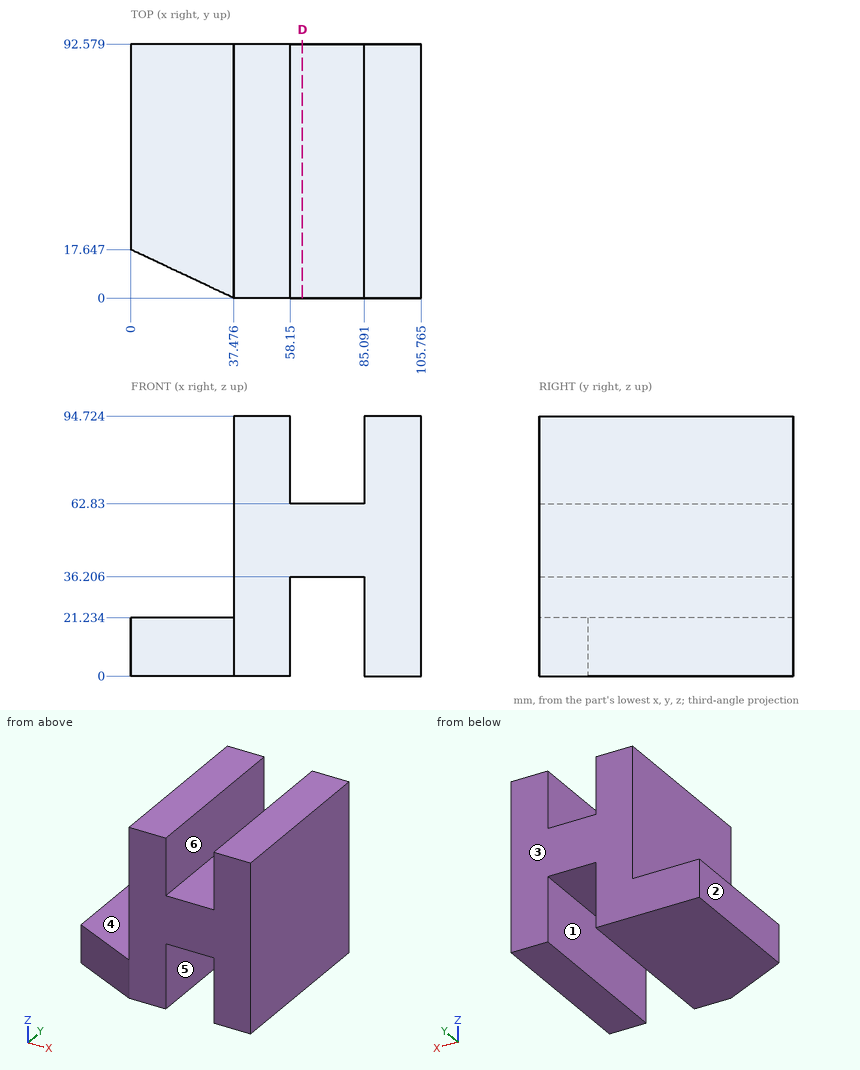
Print and shaded views of the part. All mm, measured from the part's lowest x, y and z. A direction names the side the tool comes from. Coordinates: 2 decimals unless noted, no trailing zeros. Order: outer loops, then holes, each group sorted by start corner. A loop starts at its lowest first (then second) coordinate and runs counter-clockwise, first axis right, second up. Notation, with made-up numbers: (28, -1) - (63, -1) arc R26 ccw to (63, 29) - close; hole circle Ø11 at (56.25, 43). An arc over 180 degrees is marked (long way). Return JSON: item names as keys, results as strings. Group by question number.
Item 1: Drill centre lines: probe 1 along Z at (x, y) = (58.5, 65) (1 decimal); probe 2 along X at (y, z) = (49, 55.5) (1 decimal); probe 3 along Z at (x, y) = (7.5, 83). Where is each one in solid material? Low to high. Write a range as from..to.
Item 2: Pin check, flat tips, straight feed: pin 1 (5 mm diameter, centred on y = 18.5, z = 41, fed in from -X); pin 2 (10 mm diameter, centred on x = 68.5, y = 23.5, fed in from -Z); pin 3 (13.5 mm diameter, centred on x = 66, y = 48.5, fed in from +Z). Stop position of each tip, or through.
Item 3: Which spindle directions (+Z, -Z, +X, -X, +Y, -Y) get a long thin tool onto all of the face, cutting with end or side? Do the marked faces 4, 5 and 6. Say none if no direction does.
Item 4: Pull direction X, two halves, no side cores. Call the marked faces 1, 2 and 3: pulls with the +X half, pulls with the -X half, needs draft (parallel to the pull), parting line crosses it, or undercut.
Item 5: Cut at D-D (x = 62.5). List the corners of the cut face in (y, z) (1 decimal), plus the area to 4 significant figures.
Check values:
{
 "1": {"probe 1": "z = 36.2..62.8", "probe 2": "x = 37.5..105.8", "probe 3": "z = 0..21.23"},
 "2": {"pin 1": "stops at x = 37.48", "pin 2": "stops at z = 36.21", "pin 3": "stops at z = 62.83"},
 "3": {"face 4": "+Z, -X, +Y, -Y", "face 5": "-Z, +Y, -Y", "face 6": "+Z, +Y, -Y"},
 "4": {"face 1": "undercut", "face 2": "pulls with the -X half", "face 3": "needs draft"},
 "5": {"outline": "(0, 36.2) - (92.6, 36.2) - (92.6, 62.8) - (0, 62.8) - close", "area": "2,465 mm2"}
}
